Autodesk Inventor part; units mm, degrees
ref_plane "YZ Plane" through (0, 0, 0) normal (1, 0, 0) x (0, 1, 0)
ref_plane "XZ Plane" through (0, 0, 0) normal (0, 1, 0) x (-1, 0, 0)
ref_plane "XY Plane" through (0, 0, 0) normal (0, 0, 1) x (1, 0, 0)
sketch "Sketch1" plane through (0, 0, 0) normal (0, 1, 0) x (-1, 0, 0)
  line L0 (-83.5, 139.5) -> (83.5, 139.5)
  line L1 (83.5, 139.5) -> (83.5, -139.5)
  line L2 (83.5, -139.5) -> (-83.5, -139.5)
  line L3 (-83.5, -139.5) -> (-83.5, 139.5)
  line L4 (-83.5, 139.5) -> (83.5, -139.5) construction
  line L5 (83.5, 139.5) -> (-83.5, -139.5) construction
  point P0 (0, 0)
  dimension "d0" = 167
  dimension "d1" = 279
extrude "Extrusion1" add sketch "Sketch1" along normal blind 26.6
sketch "Sketch2" plane through (0, 26.6, 0) normal (0, 1, 0) x (1, 0, 0)
  line L0 (71.5, -119.5) -> (-71.5, -119.5)
  line L1 (-73.5, -117.5) -> (-73.5, 117.5)
  line L2 (-71.5, 119.5) -> (71.5, 119.5)
  line L3 (73.5, 117.5) -> (73.5, -117.5)
  line L4 (73.5, -119.5) -> (-73.5, 119.5) construction
  line L5 (-73.5, -119.5) -> (73.5, 119.5) construction
  arc A0 (-73.5, -117.5) -> (-71.5, -119.5) centre (-71.5, -117.5) ccw
  arc A1 (-71.5, 119.5) -> (-73.5, 117.5) centre (-71.5, 117.5) ccw
  arc A2 (73.5, 117.5) -> (71.5, 119.5) centre (71.5, 117.5) ccw
  arc A3 (71.5, -119.5) -> (73.5, -117.5) centre (71.5, -117.5) ccw
  point P0 (0, 0)
  dimension "d4" = 147
  dimension "d5" = 239
  dimension "d6" = 2
extrude "Extrusion2" cut sketch "Sketch2" against normal blind 1.1
sketch "Sketch3" plane through (0, 25.5, 0) normal (0, 1, 0) x (1, 0, 0)
  line L0 (-73.5, -117.5) -> (-73.5, 117.5)
  line L1 (71.5, -119.5) -> (-71.5, -119.5)
  line L2 (-72.25, -117.83) -> (72.25, -117.83)
  line L3 (72.25, -117.83) -> (72.25, 112.27)
  line L4 (72.25, 112.27) -> (-72.25, 112.27)
  line L5 (-72.25, 112.27) -> (-72.25, -117.83)
  point P0 (0, 0)
  dimension "d9" = 1.25
  dimension "d10" = 1.67
  dimension "d11" = 144.5
  dimension "d12" = 230.1
extrude "Extrusion3" cut sketch "Sketch3" against normal blind 20
sketch "Sketch4" plane through (0, 5.5, 0) normal (0, 1, 0) x (1, 0, 0)
  circle A0 centre (-66.5, -111.83) radius 2
  line L0 (72.25, -117.83) -> (-72.25, -117.83)
  line L1 (-72.25, -117.83) -> (-72.25, 112.27)
  circle A1 centre (66.5, -111.83) radius 2
  line L2 (72.25, 112.27) -> (72.25, -117.83)
  circle A2 centre (-66.5, 106.27) radius 2
  line L3 (-72.25, 112.27) -> (72.25, 112.27)
  circle A3 centre (66.5, 106.27) radius 2
  point P0 (0, 0)
  dimension "d15" = 4
  dimension "d16" = 6
  dimension "d17" = 5.75
  dimension "d18" = 4
  dimension "d19" = 6
  dimension "d20" = 5.75
  dimension "d21" = 4
  dimension "d22" = 5.75
  dimension "d23" = 6
  dimension "d24" = 4
  dimension "d25" = 6
  dimension "d26" = 5.75
extrude "Extrusion4" add sketch "Sketch4" along normal blind 10.3 contours A0 | A1 | A2 | A3
sketch "Sketch5" plane through (0, 5.5, 0) normal (0, 1, 0) x (1, 0, 0)
  circle A0 centre (-66.5, -111.83) radius 2
  circle A1 centre (-66.5, -111.83) radius 1.25
  circle A2 centre (-66.5, 106.27) radius 2
  circle A3 centre (-66.5, 106.27) radius 1.25
  circle A4 centre (66.5, 106.27) radius 2
  circle A5 centre (66.5, 106.27) radius 1.25
  circle A6 centre (66.5, -111.83) radius 1.25
  point P0 (0, 0)
  dimension "d29" = 2.5
  dimension "d30" = 2.5
  dimension "d31" = 2.5
  dimension "d32" = 2.5
extrude "Extrusion5" cut sketch "Sketch5" along normal blind 10.3 and the other way blind 5.5 contours A1 | A3 | A5 | A6
sketch "Sketch8" plane through (0, 0, 0) normal (0, -1, 0) x (1, 0, 0)
  circle A0 centre (66.5, 111.83) radius 1.25
  circle A1 centre (66.5, 111.83) radius 1.75
  circle A2 centre (66.5, -106.27) radius 1.25
  circle A3 centre (66.5, -106.27) radius 1.75
  circle A4 centre (-66.5, -106.27) radius 1.25
  circle A5 centre (-66.5, -106.27) radius 1.75
  circle A6 centre (-66.5, 111.83) radius 1.75
  point P0 (0, 0)
  dimension "d49" = 3.5
  dimension "d50" = 3.5
  dimension "d51" = 3.5
  dimension "d52" = 3.5
extrude "Extrusion8" cut sketch "Sketch8" against normal blind 13.8
sketch "Sketch9" plane through (0, 5.5, 0) normal (0, 1, 0) x (1, 0, 0)
  line L0 (60, -100) -> (-60, -100)
  line L1 (-60, -100) -> (-60, 100)
  line L2 (-60, 100) -> (60, 100)
  line L3 (60, 100) -> (60, -100)
  line L4 (60, -100) -> (-60, 100) construction
  line L5 (-60, -100) -> (60, 100) construction
  point P0 (0, 0)
  dimension "d55" = 120
  dimension "d56" = 200
extrude "Extrusion9" cut sketch "Sketch9" against normal blind 5.8
sketch "Sketch10" plane through (0, 0, 0) normal (0, -1, 0) x (1, 0, 0)
  line L0 (83.5, 139.5) -> (83.5, -139.5)
  line L1 (-83.5, -139.5) -> (-83.5, 139.5)
  line L2 (83.5, 139.5) -> (-83.5, 139.5)
  line L3 (-83.5, 139.5) -> (-83.5, -139.5)
  line L4 (-83.5, -139.5) -> (83.5, -139.5)
  line L5 (83.5, -139.5) -> (83.5, 139.5)
  line L6 (72.25, -115.05) -> (-72.25, -115.05)
  line L7 (-72.25, -115.05) -> (-72.25, 115.05)
  line L8 (-72.25, 115.05) -> (72.25, 115.05)
  line L9 (72.25, 115.05) -> (72.25, -115.05)
  line L10 (72.25, -115.05) -> (-72.25, 115.05) construction
  line L11 (-72.25, -115.05) -> (72.25, 115.05) construction
  line L12 (-83.5, -139.5) -> (83.5, -139.5)
  line L13 (83.5, -139.5) -> (83.5, 139.5)
  line L14 (83.5, 139.5) -> (-83.5, 139.5)
  line L15 (-83.5, 139.5) -> (-83.5, -139.5)
  point P0 (0, 0)
  point P1 (71.5, 119.5)
  dimension "d67" = 144.5
  dimension "d68" = 230.1
extrude "Extrusion10" add sketch "Sketch10" along normal blind 40
sketch "Sketch12" plane through (0, -40, 0) normal (0, -1, 0) x (1, 0, 0)
  line L0 (-72.25, -115.05) -> (-72.25, 115.05)
  line L1 (72.25, -115.05) -> (-72.25, -115.05)
  line L2 (-77.25, -120.05) -> (-72.25, -120.05)
  line L3 (-72.25, -120.05) -> (-72.25, 120.05)
  line L4 (-72.25, 120.05) -> (-77.25, 120.05)
  line L5 (-77.25, 120.05) -> (-77.25, -120.05)
  line L6 (72.25, 115.05) -> (72.25, -115.05)
  line L7 (77.25, -120.05) -> (72.25, -120.05)
  line L8 (72.25, -120.05) -> (72.25, 120.05)
  line L9 (72.25, 120.05) -> (77.25, 120.05)
  line L10 (77.25, 120.05) -> (77.25, -120.05)
  line L11 (72.25, 115.05) -> (-72.25, 115.05)
  line L12 (72.25, 120.05) -> (-72.25, 120.05)
  line L13 (-72.25, 120.05) -> (-72.25, 115.05)
  line L14 (-72.25, 115.05) -> (72.25, 115.05)
  line L15 (72.25, 115.05) -> (72.25, 120.05)
  line L16 (-83.5, 139.5) -> (-83.5, -139.5)
  line L17 (83.5, 139.5) -> (-83.5, 139.5)
  line L18 (-83.5, -139.5) -> (83.5, -139.5)
  line L19 (83.5, -139.5) -> (83.5, 139.5)
  line L20 (83.5, 139.5) -> (-83.5, 139.5)
  line L21 (-83.5, 139.5) -> (-83.5, -139.5)
  line L22 (-72.25, -115.05) -> (72.25, -115.05)
  line L23 (-72.25, -115.05) -> (72.25, -115.05)
  line L24 (72.25, -115.05) -> (72.25, -120.05)
  line L25 (72.25, -120.05) -> (-72.25, -120.05)
  line L26 (-72.25, -120.05) -> (-72.25, -115.05)
  point P0 (0, 0)
  dimension "d69" = 5
  dimension "d70" = 5
  dimension "d71" = 240.1
  dimension "d72" = 5
  dimension "d73" = 5
  dimension "d74" = 240.1
extrude "Extrusion11" add sketch "Sketch12" along normal blind 10
sketch "Sketch13" plane through (0, -50, 0) normal (0, -1, 0) x (1, 0, 0)
  circle A0 centre (-77.5, -133.5) radius 1.25
  line L0 (-83.5, 139.5) -> (-83.5, -139.5)
  line L1 (-83.5, -139.5) -> (83.5, -139.5)
  circle A1 centre (-77.5, 133.5) radius 1.25
  line L2 (83.5, 139.5) -> (-83.5, 139.5)
  circle A2 centre (77.5, 133.5) radius 1.25
  line L3 (83.5, -139.5) -> (83.5, 139.5)
  circle A3 centre (77.5, -133.5) radius 1.25
  point P0 (0, 0)
  dimension "d77" = 2.5
  dimension "d78" = 6
  dimension "d79" = 6
  dimension "d80" = 2.5
  dimension "d81" = 6
  dimension "d82" = 6
  dimension "d83" = 2.5
  dimension "d84" = 6
  dimension "d85" = 6
  dimension "d86" = 6
  dimension "d87" = 6
extrude "Extrusion12" cut sketch "Sketch13" against normal blind 10 contours A0 | A1 | A2 | A3
properties part number "Enclosure"
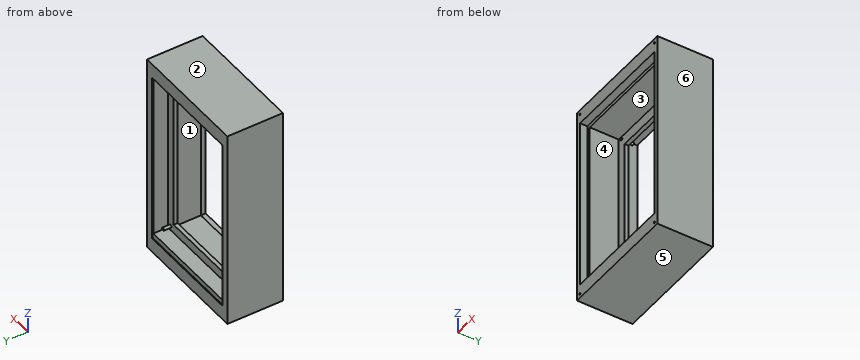
The model under review builds one solid part; all positions refer to its coordinate system, in mm. Face numbers are marked on the shaded views. A direction names the side the tool comes from. Round coordinates to 2 decimals unless told otherwise and drop trailing zeros. Order: outer loops, then holes, each group sorted by start corner. A loop starts at its lowest first (then second) coordinate and runs counter-clockwise, first axis right, second up. Notation, with made-up numbers: (68.25, 31.5) -> (82.25, 31.5) arc R19 ccw to (82.25, 61.5) -> close; hole circle Ø11 at (49.5, 16.25). An arc over 180 degrees is marked (long way). Write item = value, one per line. Start each with the question number.
Item 1: Mouldability with a two-part tool opening along X and no side actions: class the marked faces 3, 4, 5 and 6 as released by +X, released by -X, zero draft, split by the parting line, or undercut.
Item 2: Consider section A-A on z = -3. Write out the cut boundary in (x, y), plus the area to 3 significant figures.
Item 3: For line 1 along X through (y, z) = (6, -106.27); line 2 along X through (y, z) = (-42.75, -133.5); line 3 along X through (y, z) = (14.9, -106.27), list the stretches that pass through material, from the lowest coordinate up.
Item 4: For the marked faces 1 and 2, list the 3-axis set-ups (+Z, -Z, +X, -X, +Y, -Y) from which the entire face can be reached by the end or side of a thin tool; tool diameter is ignored.
Item 5: Consider section C-C on y = 21. Write out the cut boundary in (x, z).
Item 6: Clearance check with flat-ended pins moving along their axes: pin 1 Ø3 at (x, z) = (65.5, 111.5) entering from +Y; pin 2 Ø1 at (x, z) = (26, 102.5) entering from -Y; pin 3 Ø1.2 at (x, z) = (-77.5, 134) entering from -Y. State where each tip first meets the part, or that it passes through.
Item 7: Consider section B-B on x = -10.5. Write out the cut boundary in (y, z), plus the area to 3 significant figures.
Conclusion:
q1.face_3 = undercut
q1.face_4 = undercut
q1.face_5 = zero draft
q1.face_6 = released by +X
q2.outline = (-83.5, -50) -> (-77.25, -50) -> (-77.25, -40) -> (-72.25, -40) -> (-72.25, 0) -> (-60, 0) -> (-60, 5.5) -> (-72.25, 5.5) -> (-72.25, 25.5) -> (-73.5, 25.5) -> (-73.5, 26.6) -> (-83.5, 26.6) -> close; (60, 0) -> (72.25, 0) -> (72.25, -40) -> (77.25, -40) -> (77.25, -50) -> (83.5, -50) -> (83.5, 26.6) -> (73.5, 26.6) -> (73.5, 25.5) -> (72.25, 25.5) -> (72.25, 5.5) -> (60, 5.5) -> close
q2.area = 1,760 mm2
q3.line_1 = -83.5 to -72.25, -68.5 to -68.25, -64.75 to -64.5, 64.5 to 64.75, 68.25 to 68.5, 72.25 to 83.5
q3.line_2 = -83.5 to -78.75, -76.25 to 76.25, 78.75 to 83.5
q3.line_3 = -83.5 to -72.25, -68.5 to -67.75, -65.25 to -64.5, 64.5 to 65.25, 67.75 to 68.5, 72.25 to 83.5
q4.face_1 = -Y
q4.face_2 = +Z, +X, -X, +Y, -Y
q5.outline = (-83.5, -139.5) -> (83.5, -139.5) -> (83.5, 139.5) -> (-83.5, 139.5) -> close; hole (-72.25, -112.27) -> (72.25, -112.27) -> (72.25, 117.83) -> (-72.25, 117.83) -> close
q6.pin_1 = 15.8
q6.pin_2 = 0
q6.pin_3 = -40
q7.outline = (-50, -139.5) -> (26.6, -139.5) -> (26.6, -119.5) -> (25.5, -119.5) -> (25.5, -112.27) -> (5.5, -112.27) -> (5.5, -100) -> (0, -100) -> (0, -115.05) -> (-40, -115.05) -> (-40, -120.05) -> (-50, -120.05) -> close; (-50, 120.05) -> (-40, 120.05) -> (-40, 115.05) -> (0, 115.05) -> (0, 100) -> (5.5, 100) -> (5.5, 117.83) -> (25.5, 117.83) -> (25.5, 119.5) -> (26.6, 119.5) -> (26.6, 139.5) -> (-50, 139.5) -> close
q7.area = 3,800 mm2
